Check sheet for the modelled part. Datum: model origin and axes. Units: mm. Face numbers are marked on the shaded views. A direction names the side the tool comes from. Round coordinates to 2 decimals unless told otherwise and drop trailing zeros. Write each loop counter-clockwise with the first axis right and the second up, starting at its lowest first coordinate (ties: lowest second). Pieces come first, ordered by that corner, then holes. Notation, with made-up numbers: (-35, 37) -> (19, 37) arc R10 ccw to (19, 46) -> close; hole circle Ø7 at (79, 86.5). An arc over 180 degrees is marked (long way). One line per item, written item: value. Start each with the question number.
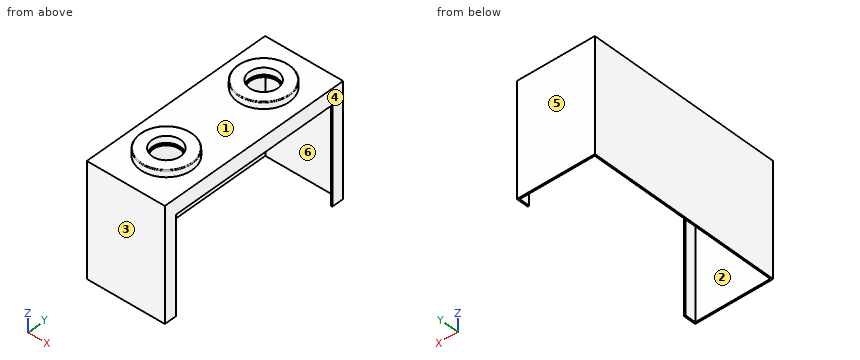
```python
from build123d import *

# Parameters (mm, degrees)
F0_W     = 104
F0_H     = 151
F1_DEPTH = 262
F2_T     = -2
F3_W     = 230
F3_H     = 130
F4_DEPTH = 2
F5_R     = 17.5
F6_DEPTH = 25
F7_R     = 34.5
F7_R_2   = 19
F8_DEPTH = 9
F9_R     = 1


with BuildPart() as f1:
    # F0 (on Front) → F1 (new body)
    with BuildSketch(Plane.XZ):
        with Locations((52, 75.5)):
            Rectangle(F0_W, F0_H)
    extrude(amount=F1_DEPTH)

    # F2
    f2_openings = [f1.faces().sort_by_distance(p)[0] for p in [
        (52, -131, 0),
    ]]
    offset(amount=F2_T, openings=f2_openings)

    # F3 (on face) → F4 (cut, through all)
    with BuildSketch(Plane.YZ.offset(104)):
        with Locations((-131, 65)):
            Rectangle(F3_W, F3_H)
    extrude(amount=-F4_DEPTH, mode=Mode.SUBTRACT)

    # F5 (on face) → F6 (cut)
    with BuildSketch(Plane.XY.offset(151)):
        with Locations((52, -59.5)):
            Circle(F5_R)
        with Locations((52, -202.5)):
            Circle(F5_R)
    extrude(amount=-F6_DEPTH, mode=Mode.SUBTRACT)

    # F7 (on face) → F8 (join)
    with BuildSketch(Plane.XY.offset(151)):
        with Locations((52, -59.5)):
            Circle(F7_R)
        with Locations((52, -59.5)):
            Circle(F7_R_2, mode=Mode.SUBTRACT)
        with Locations((52, -202.5)):
            Circle(F7_R)
        with Locations((52, -202.5)):
            Circle(F7_R_2, mode=Mode.SUBTRACT)
    extrude(amount=F8_DEPTH)

    # F9
    f9_edges = [f1.edges().sort_by_distance(p)[0] for p in [
        (17.5, -59.5, 160),
        (17.5, -202.5, 160),
    ]]
    fillet(f9_edges, radius=F9_R)


solid = f1.part
```
1. Depth check by flat-ended pin: pin 1 Ø1 at (x, y) = (102.5, -106.5) entering from -Z; pin 2 Ø10 at (x, y) = (80.5, -216.5) entering from -Z; pin 3 Ø19 at (x, y) = (54, -194.5) entering from +Z. Enter the tip coordinate at first touch or a pass-through.
2. Access from +Z, -Z, +X, -X, +Y, -Y to the whole of each face (thin tool, end or side, straight path). Record for the marked faces 1, 2 and 3.
3. Cross-section at A-A (y = -202.5). Record the cut outline in (x, z), plus the area to 3 significant figures.
4. Cross-section at C-C (x = 97.5). Record the cut outline in (y, z).
5. Cross-section at D-D (z = 99). Record the cut outline in (x, y), plus the area to 3 significant figures.
6. Release check for a two-part mould opening along X. For the marked faces 4, 5 and 6 record: +X half, -X half, draft (parallel to the pull), parting line (faces both ways), or undercut.
7. Cross-section at B-B (z = 138). Record the cut outline in (x, y).
8. Material ranges on probe 1 along Y at (x, z) = (52, 153.75); probe 2 along Y at (x, z) = (11, 9.5); probe 3 along X at (y, z) = (-59, 150), recorded low to high.
Working result:
1. pin 1: stops at z = 130
1. pin 2: stops at z = 149
1. pin 3: stops at z = 151
2. face 1: +Z
2. face 2: -Z
2. face 3: +Z, -Z, +X, -X, -Y
3. outline: (0, 0) -> (2, 0) -> (2, 149) -> (34.5, 149) -> (34.5, 151) -> (33, 151) -> (33, 160) -> (18.5, 160) arc R1 ccw to (17.5, 159) -> (17.5, 151) -> (0, 151) -> close; (69.5, 149) -> (102, 149) -> (102, 130) -> (104, 130) -> (104, 151) -> (86.5, 151) -> (86.5, 159) arc R1 ccw to (85.5, 160) -> (71, 160) -> (71, 151) -> (69.5, 151) -> close
3. area: 753 mm^2
4. outline: (-262, 0) -> (-260, 0) -> (-260, 149) -> (-2, 149) -> (-2, 0) -> (0, 0) -> (0, 151) -> (-262, 151) -> close
5. outline: (0, -262) -> (104, -262) -> (104, -246) -> (102, -246) -> (102, -260) -> (2, -260) -> (2, -2) -> (102, -2) -> (102, -16) -> (104, -16) -> (104, 0) -> (0, 0) -> close
5. area: 988 mm^2
6. face 4: +X half
6. face 5: draft
6. face 6: undercut
7. outline: (0, -262) -> (104, -262) -> (104, 0) -> (0, 0) -> close; hole (2, -260) -> (102, -260) -> (102, -2) -> (2, -2) -> close
8. probe 1: y = -237 to -221.5, -183.5 to -168, -94 to -78.5, -40.5 to -25
8. probe 2: y = -262 to -260, -2 to 0
8. probe 3: x = 0 to 34.51, 69.49 to 104
